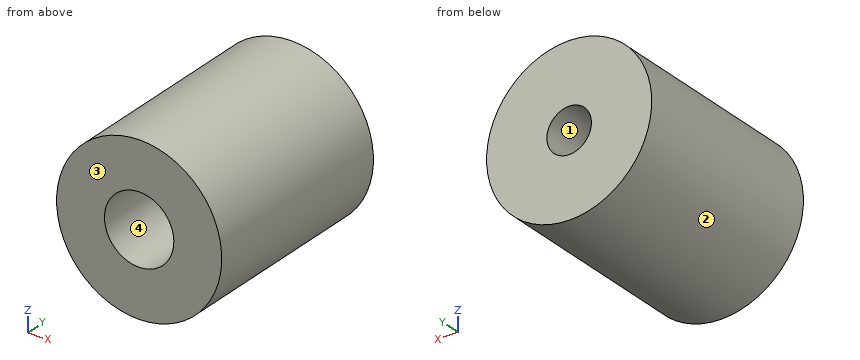
```python
from build123d import *

# Parameters (mm, degrees)
SKETCH1_R           = 10
BOSS_EXTRUDE1_DEPTH = 12.5
SKETCH2_R           = 2.7
CUT_EXTRUDE1_DEPTH  = 12.5
SKETCH3_R           = 4.2
CUT_EXTRUDE2_DEPTH  = 12.5


with BuildPart() as part:
    # Sketch1 → Boss-Extrude1 (new, symmetric)
    with BuildSketch(Plane(origin=(0, 0, 0), x_dir=(1, 0, 0), z_dir=(0, 1, 0))):
        with Locations(Location((0, 0, 0), (0, 0, 270))):
            Circle(SKETCH1_R)
    extrude(amount=BOSS_EXTRUDE1_DEPTH, both=True)

    # Sketch2 → Cut-Extrude1 (cut)
    with BuildSketch(Plane(origin=(0, 0, 0), x_dir=(1, 0, 0), z_dir=(0, 1, 0))):
        with Locations(Location((0, 0, 0), (0, 0, 270))):
            Circle(SKETCH2_R)
    extrude(amount=CUT_EXTRUDE1_DEPTH, mode=Mode.SUBTRACT)

    # Sketch3 → Cut-Extrude2 (cut)
    with BuildSketch(Plane(origin=(0, 0, 0), x_dir=(1, 0, 0), z_dir=(0, 1, 0))):
        with Locations(Location((0, 0, 0), (0, 0, 270))):
            Circle(SKETCH3_R)
    extrude(amount=-CUT_EXTRUDE2_DEPTH, mode=Mode.SUBTRACT)


solid = part.part
```
Here's how the part is built. I have some questions about the finished solid (model axes, mm). Face numbers are marked on the shaded views. Coordinates: 2 decimals unless noted, no trailing zeros. Write each loop counter-clockwise with the first axis right and the second up, starting at its lowest first coordinate (ties: lowest second). Pieces come first, ordered by that corner, then holes. Notation, with made-up numbers: (-3, 51.25) - (14, 51.25) arc R24 cw to (14, 64.25) - close; hole circle Ø4 at (16.5, 50). An arc over 180 degrees is marked (long way). One line per item, written item: value.
1) I'm going to push flat-ended pins straight in: P1, Ø2, axis at y = -1, z = 6.5, coming from the -X side; P2, Ø1, axis at x = 3, y = -9.5, coming from the -Z side; P3, Ø10, axis at y = 2.5, z = -6, coming from the +X side. Where does each tip first touch, or does it pass through?
Model answer:
P1: stops at x = -8.35
P2: stops at z = -9.68
P3: stops at x = 9.95
2) Suppose I cut it at B-B on z = 0. Write out the boundary of the cut face in (x, y).
Model answer:
outline: (-10, -12.5) - (-4.2, -12.5) - (-4.2, 0) - (-2.7, 0) - (-2.7, 12.5) - (-10, 12.5) - close; (2.7, 0) - (4.2, 0) - (4.2, -12.5) - (10, -12.5) - (10, 12.5) - (2.7, 12.5) - close
3) I need wall thicknesses on line 1 along X through (y, z) = (8, 0); line 2 along X through (y, z) = (-6.5, 0); line 3 along Z through (x, y) = (-1.5, 6.25) (3 decimals). Which ranges of each line are inside material? Lowest first, please.
Model answer:
line 1: x = -10 to -2.7, 2.7 to 10
line 2: x = -10 to -4.2, 4.2 to 10
line 3: z = -9.887 to -2.245, 2.245 to 9.887
4) Suppose I cut it at D-D on y = 10.75. Write out the boundary of the cut face in (x, z).
Model answer:
outline: circle Ø20 at (0, 0); hole circle Ø5.4 at (0, 0)
5) Suppose I cut it at A-A on x = 0. Write out the boundary of the cut face in (y, z).
Model answer:
outline: (-12.5, -10) - (12.5, -10) - (12.5, -2.7) - (0, -2.7) - (0, -4.2) - (-12.5, -4.2) - close; (-12.5, 4.2) - (0, 4.2) - (0, 2.7) - (12.5, 2.7) - (12.5, 10) - (-12.5, 10) - close
6) Suppose I cut it at C-C on y = -9.75. Write out the boundary of the cut face in (x, z), and give its area (3 significant figures).
Model answer:
outline: circle Ø20 at (0, 0); hole circle Ø8.4 at (0, 0)
area: 259 mm²
7) We'd pull the mould along X, two halves only. Please class the marked faces 1, 2, 3 and 4: pulls with the +X half, pulls with the -X half, needs draft (parallel to the pull), parting line crosses it, or undercut.
Model answer:
face 1: undercut
face 2: parting line crosses it
face 3: needs draft
face 4: undercut
